Design review of the part built by this model. Coordinates are the model's own, in mm. Give positions to 0.01 mm unless a question says otherwise; leave off trailing zeros. Write each loop counter-clockwise with the first axis right and the second up, starting at its lowest first coordinate (ties: lowest second). Pieces come first, ordered by that corner, then holes. Notation, with made-up numbers: (59.25, 19) - (108.25, 19) arc R30 cw to (108.25, 57) - close; hole circle Ø4 at (64, 15.25). An arc over 180 degrees is marked (long way). Use a Markdown table: item, result. Add a question column.
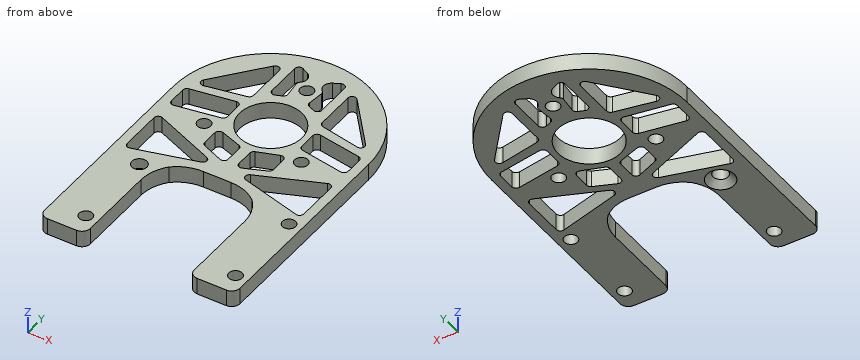
```python
from build123d import *

# Parameters (mm, degrees)
SKETCH_1_R                   = 1.6
SKETCH_1_R_2                 = 7.5
EXTRUDE_1_DEPTH              = 4
SKETCH_2_R                   = 1.6
CUT_EXTRUDE_1_DEPTH          = 56.391786395
CUT_EXTRUDE_2_DEPTH          = 56.391786395
FILLET_2_R                   = 10
FILLET_3_R                   = 2
CUT_EXTRUDE_3_DEPTH          = 56.391786395
FILLET_4_R                   = 2
FILLET_5_R                   = 1
HOLE_WIZARD_M3_1_D           = 3.6
HOLE_WIZARD_M3_1_CSINK_D     = 6.6
HOLE_WIZARD_M3_1_CSINK_ANGLE = 90


with BuildPart() as part:
    # 草图1 → 凸台-拉伸1 (new body)
    with BuildSketch(Plane.XY):
        with BuildLine():
            Line((-23.5, 0), (-23.5, -50))
            Line((-23.5, -50), (23.5, -50))
            Line((23.5, -50), (23.5, 0))
            ThreePointArc((23.5, 0), (0, 23.5), (-23.5, 0))
        make_face()
        with Locations((0, 13.5)):
            Circle(SKETCH_1_R, mode=Mode.SUBTRACT)
        with Locations((11.691342951, -6.75)):
            Circle(SKETCH_1_R, mode=Mode.SUBTRACT)
        with Locations((-11.691342951, -6.75)):
            Circle(SKETCH_1_R, mode=Mode.SUBTRACT)
        Circle(SKETCH_1_R_2, mode=Mode.SUBTRACT)
    extrude(amount=EXTRUDE_1_DEPTH)

    # 草图2 → 切除-拉伸1 (cut, through all)
    with BuildSketch(Plane.XY.offset(4)):
        with Locations((20.5, -45)):
            Circle(SKETCH_2_R)
        with Locations((20.5, -25)):
            Circle(SKETCH_2_R)
        with Locations((-15.5, -45)):
            Circle(SKETCH_2_R)
        with Locations((-15.5, -25)):
            Circle(SKETCH_2_R)
    extrude(amount=-CUT_EXTRUDE_1_DEPTH, mode=Mode.SUBTRACT)

    # 草图3 → 切除-拉伸2 (cut, through all)
    with BuildSketch(Plane.XY.offset(4)):
        Polygon((12.5, -25), (7.5, -20), (-7.5, -20), (-12.5, -25), (-12.5, -50), (12.5, -50), align=None)
    extrude(amount=-CUT_EXTRUDE_2_DEPTH, mode=Mode.SUBTRACT)

    # 圆角2
    # the kernel refuses this fillet: 10 mm, written as the material it adds along each edge
    with BuildSketch(Plane(origin=(-12.5, -25, 4), x_dir=(0, -1, 0), z_dir=(0, 0, -1))) as fillet_2_piece_1:
        with BuildLine():
            CenterArc((FILLET_2_R * 0.414213562373, -FILLET_2_R), FILLET_2_R, 90, 45)
            Line((-FILLET_2_R * 0.292893218813, -FILLET_2_R * 0.292893218813), (0, 0))
            Line((0, 0), (FILLET_2_R * 0.414213562373, 0))
        make_face()
    extrude(amount=4)
    with BuildSketch(Plane(origin=(-7.5, -20, 4), x_dir=(1, 0, 0), z_dir=(0, 0, -1)), Plane(origin=(7.5, -20, 4), x_dir=(0.7071067811865472, -0.7071067811865479, 0), z_dir=(0, 0, -1)), Plane(origin=(12.5, -25, 4), x_dir=(0, -1, 0), z_dir=(0, 0, -1))) as fillet_2_piece_2:
        with BuildLine():
            CenterArc((FILLET_2_R * 0.414213562373, FILLET_2_R), FILLET_2_R, 225, 45)
            Line((-FILLET_2_R * 0.292893218813, FILLET_2_R * 0.292893218813), (0, 0))
            Line((0, 0), (FILLET_2_R * 0.414213562373, 0))
        make_face()
    extrude(amount=4)

    # 圆角3
    fillet_3_edges = [part.edges().sort_by_distance(p)[0] for p in [
        (-12.5, -50, 2),
        (12.5, -50, 2),
        (23.5, -50, 2),
        (-23.5, -50, 2),
    ]]
    fillet(fillet_3_edges, radius=FILLET_3_R)

    # 草图4 → 切除-拉伸3 (cut, through all)
    with BuildSketch(Plane.XY.offset(4)):
        Polygon((8.242977091, 18.793122214), (21.245983207, 3.003757645), (8.242977091, 5.544260941), align=None)
        Polygon((5.998410559, 19.876706057), (5.998410559, 8.266879168), (2.515462493, 9.660058395), (3.057254414, 14.69098338), (0.503092499, 17.090347604), align=None)
        Polygon((21.245983207, 0.953850638), (21.245983207, -5.286408991), (8.939449972, -3.17573294), (8.939449972, 3.003757645), align=None)
        Polygon((21.245983207, -9.127756299), (21.245983207, -21.963810312), (2.515462493, -16.865803044), align=None)
        Polygon((8.242977091, -6.687008394), (8.242977091, -12.519465541), (1.285419198, -15.393806785), (1.285419198, -9.127756299), align=None)
        Polygon((-3.057254414, 14.69098338), (-0.503092499, 17.090347604), (-5.998410559, 19.876706057), (-5.998410559, 8.266879168), (-2.515462493, 9.660058395), align=None)
        Polygon((-21.245983207, 3.003757645), (-8.242977091, 5.544260941), (-8.242977091, 18.793122214), align=None)
        Polygon((-8.939449972, -3.17573294), (-8.939449972, 3.003757645), (-21.245983207, 0.953850638), (-21.245983207, -5.286408991), align=None)
        Polygon((-21.245983207, -21.963810312), (-2.515462493, -16.865803044), (-21.245983207, -9.127756299), align=None)
        Polygon((-1.285419198, -15.393806785), (-1.285419198, -9.127756299), (-8.242977091, -6.687008394), (-8.242977091, -12.519465541), align=None)
    extrude(amount=-CUT_EXTRUDE_3_DEPTH, mode=Mode.SUBTRACT)

    # 圆角4
    fillet_4_edges = [part.edges().sort_by_distance(p)[0] for p in [
        (0.503092499, 17.090347604, 2),
        (-0.503092499, 17.090347604, 2),
    ]]
    fillet(fillet_4_edges, radius=FILLET_4_R)

    # 圆角5
    fillet_5_edges = [part.edges().sort_by_distance(p)[0] for p in [
        (5.998410559, 19.876706057, 2),
        (5.998410559, 8.266879168, 2),
        (2.515462493, 9.660058395, 2),
        (3.057254414, 14.69098338, 2),
        (8.939449972, 3.003757645, 2),
        (21.245983207, 0.953850638, 2),
        (21.245983207, -5.286408991, 2),
        (8.939449972, -3.17573294, 2),
        (1.285419198, -9.127756299, 2),
        (8.242977091, -6.687008394, 2),
        (8.242977091, -12.519465541, 2),
        (1.285419198, -15.393806785, 2),
        (2.515462493, -16.865803044, 2),
        (21.245983207, -9.127756299, 2),
        (21.245983207, -21.963810312, 2),
        (-21.245983207, -21.963810312, 2),
        (-21.245983207, -9.127756299, 2),
        (-2.515462493, -16.865803044, 2),
        (-8.939449972, -3.17573294, 2),
        (-21.245983207, -5.286408991, 2),
        (-21.245983207, 0.953850638, 2),
        (-8.939449972, 3.003757645, 2),
        (-21.245983207, 3.003757645, 2),
        (-8.242977091, 18.793122214, 2),
        (-8.242977091, 5.544260941, 2),
        (-3.057254414, 14.69098338, 2),
        (-2.515462493, 9.660058395, 2),
        (-5.998410559, 8.266879168, 2),
        (-5.998410559, 19.876706057, 2),
        (-1.285419198, -15.393806785, 2),
        (-8.242977091, -12.519465541, 2),
        (-8.242977091, -6.687008394, 2),
        (-1.285419198, -9.127756299, 2),
        (8.242977091, 5.544260941, 2),
        (8.242977091, 18.793122214, 2),
        (21.245983207, 3.003757645, 2),
    ]]
    fillet(fillet_5_edges, radius=FILLET_5_R)

    # M3 十字槽半沉头木螺钉的锥形沉头孔1 (through all)
    with Locations(Plane(origin=(0, 0, 0), x_dir=(-1, 0, 0), z_dir=(0, 0, -1))):
        with Locations((15.5, -25)):
            CounterSinkHole(HOLE_WIZARD_M3_1_D / 2, HOLE_WIZARD_M3_1_CSINK_D / 2, counter_sink_angle=HOLE_WIZARD_M3_1_CSINK_ANGLE)


solid = part.part
```
(1) For line 1 along X through (y, z) = (-16.5, 2.35); line 2 along Y through (x, z) = (0, 1.85); line 3 along Y through (x, z) = (-19.5, 3), list the stretches that pass through material, from the lowest coordinate up.
(2) Add section A-A (x = 0). State the section outline as (y, z) points, and give its area (3 significant figures).
(3) Insertion check: pin 1 (1.2 mm diameter, centred on y = 13.5, z = 2.5, fed in from -X); pin 2 (1.2 mm diameter, centred on x = 1.5, z = 2, fed in from -Y). Each pin has a flat end and moves straight along its axis. Give the tip position at first contact, or say it passes through.
(4) Add section D-D (z = 3.25). Count the separate pieces of the cut face and the enclosed holes in it, and give its area (3 significant figures).
(5) Add section C-C (x = -15.5). State the section outline as (y, z) points, and give its area (3 significant figures).
(6) Add section B-B (y = -45). State the section outline as (x, z) points.
Answers follow:
| question | item | result |
|---|---|---|
| 1 | line 1 | -23.5 to -21.25, -4.62 to 4.62, 21.25 to 23.5 |
| 1 | line 2 | -20 to -7.5, 7.5 to 11.9, 15.1 to 23.5 |
| 1 | line 3 | -50 to -21.49, -9.85 to -4.99, 1.24 to 3.92, 5.12 to 13.11 |
| 2 | outline | (-20, 0) - (-7.5, 0) - (-7.5, 4) - (-20, 4) - close; (7.5, 0) - (11.9, 0) - (11.9, 4) - (7.5, 4) - close; (15.1, 0) - (23.5, 0) - (23.5, 4) - (15.1, 4) - close |
| 2 | area | 101 mm^2 |
| 3 | pin 1 | x = -19.64 |
| 3 | pin 2 | y = -20 |
| 4 | separate pieces | 1 |
| 4 | enclosed holes | 18 |
| 4 | area | 1,560 mm^2 |
| 5 | outline | (-50, 0) - (-46.6, 0) - (-46.6, 4) - (-50, 4) - close; (-43.4, 0) - (-28.3, 0) - (-26.8, 1.5) - (-26.8, 4) - (-43.4, 4) - close; (-23.2, 1.5) - (-21.7, 0) - (-20.4, 0) - (-20.4, 4) - (-23.2, 4) - close; (-11.5, 0) - (-4.3, 0) - (-4.3, 4) - (-11.5, 4) - close; (1.91, 0) - (4.13, 0) - (4.13, 4) - (1.91, 4) - close; (9.98, 0) - (17.66, 0) - (17.66, 4) - (9.98, 4) - close |
| 5 | area | 157 mm^2 |
| 6 | outline | (-23.5, 0) - (-17.1, 0) - (-17.1, 4) - (-23.5, 4) - close; (-13.9, 0) - (-12.5, 0) - (-12.5, 4) - (-13.9, 4) - close; (12.5, 0) - (18.9, 0) - (18.9, 4) - (12.5, 4) - close; (22.1, 0) - (23.5, 0) - (23.5, 4) - (22.1, 4) - close |
